The listing builds one solid part. Answer for the finished solid, in the listing's coordinates (mm). Face numbers are marked on the shaded views. A direction names the side the tool comes from. Give positions to 0.01 mm unless a question says otherwise; leave off trailing zeros. Loops run counter-clockwise (first coordinate to the right, second up) from the corner with the lowest first, then second, coordinate; pieces in that order, holes last. Notation, with made-up numbers: (33, -19) - (76, -19) arc R20 cw to (76, -7) - close; hole circle Ø8 at (74.25, 37.5). An arc over 180 degrees is marked (long way). Write each question's results on one line, items separated by ' | '.
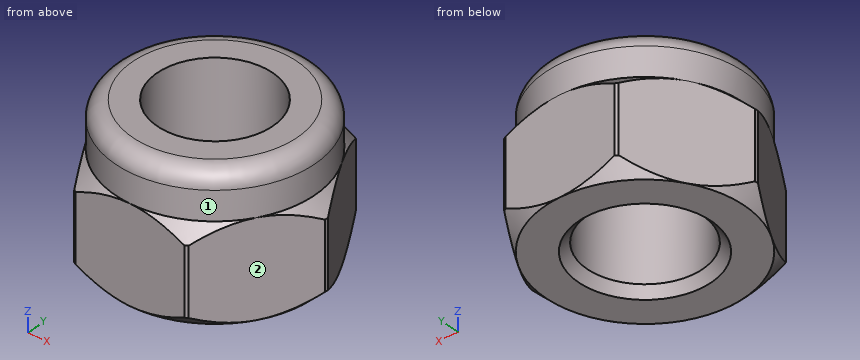
from build123d import *

# Parameters (mm, degrees)
SKETCH1_R           = 2
BOSS_EXTRUDE1_DEPTH = 3.3
SKETCH2_R           = 3.45
SKETCH2_R_2         = 2
BOSS_EXTRUDE2_DEPTH = 1.6
FILLET1_R           = 0.6
CHAMFER1_SIZE       = 0.3


with BuildPart() as part:
    # Sketch1 → Boss-Extrude1 (new body)
    with BuildSketch(Plane.XY):
        Polygon((-1.991858429, 3.45), (1.991858429, 3.45), (3.983716857, 0), (1.991858429, -3.45), (-1.991858429, -3.45), (-3.983716857, 0), align=None)
        Circle(SKETCH1_R, mode=Mode.SUBTRACT)
    extrude(amount=BOSS_EXTRUDE1_DEPTH)

    # Sketch2 → Boss-Extrude2 (add)
    with BuildSketch(Plane.XY.offset(3.3)):
        Circle(SKETCH2_R)
        Circle(SKETCH2_R_2, mode=Mode.SUBTRACT)
    extrude(amount=BOSS_EXTRUDE2_DEPTH)

    # Fillet1
    fillet1_edges = [part.edges().sort_by_distance(p)[0] for p in [
        (-3.45, 0, 4.9),
    ]]
    fillet(fillet1_edges, radius=FILLET1_R)

    # Sketch3 → Cut-Revolve1 (revolve, cut)
    with BuildSketch(Plane(origin=(0, 0, 0), x_dir=(0, 0, -1), z_dir=(1, 0, 0))):
        Polygon((-3.3, 3.45), (-2.814276913, 3.95), (-0.485723087, 3.95), (0, 3.45), (0, 4.719262328), (-3.3, 4.719262328), align=None)
    revolve(axis=Axis((0, 0, 0), (0, 0, -1)), mode=Mode.SUBTRACT)

    # Chamfer1
    chamfer1_edges = [part.edges().sort_by_distance(p)[0] for p in [
        (-2, 0, 0),
    ]]
    chamfer(chamfer1_edges, length=CHAMFER1_SIZE)


solid = part.part
Item 1: A cutting plane is placed at A-A, the plane z = 3.15. Determine the outline of the cut face in (x, y).
Values found:
outline: (-3.51, -0.82) - (-2.47, -2.63) arc R3.6 ccw to (-1.04, -3.45) - (1.04, -3.45) arc R3.6 ccw to (2.47, -2.63) - (3.51, -0.82) arc R3.6 ccw to (3.51, 0.82) - (2.47, 2.63) arc R3.6 ccw to (1.04, 3.45) - (-1.04, 3.45) arc R3.6 ccw to (-2.47, 2.63) - (-3.51, 0.82) arc R3.6 ccw to start; hole circle Ø4 at (0, 0)
Item 2: Flat-ended cylindrical pins translate along their axes: P1, Ø2, axis at y = -1.5, z = 2, coming from the +X side; P2, Ø1.5, axis at y = -1.5, z = 3.5, coming from the +X side. Find the tip coordinate at first contact, or state that the pin passes through.
Values found:
P1: stops at x = 3.7 | P2: stops at x = 3.5
Item 3: Find the intervals of material crossed by line 1 along Y through (x, z) = (0, 3.4); line 2 along X through (y, z) = (0.75, 3.5), in increasing order. Write a range as [from, to].
Values found:
line 1: y = [-3.45, -2], [2, 3.45] | line 2: x = [-3.37, -1.85], [1.85, 3.37]
Item 4: For the marked faces 1 and 2, determine the directions among +Z, -Z, +X, -X, +Y, -Y from which every point of the face is accessible in a straight line to the end or side of a thin tool.
Values found:
face 1: +Z | face 2: +Z, -Z, +X, -Y
